Input: part model. Units: mm. Frame: model coordinates. Face numbers are marked on the shaded views. A direction names the side the tool comes from. Coordinates: 2 decimals unless noted, no trailing zeros. Order: outer loops, then holes, each group sorted by start corner. A loop starts at its lowest first (then second) coordinate and runs counter-clockwise, first axis right, second up.
from build123d import *

# Parameters (mm, degrees)
BOSS_EXTRUDE1_DEPTH = 54
BOSS_EXTRUDE2_DEPTH = 1.5
SKETCH3_W           = 2.3
SKETCH3_H           = 3
CUT_EXTRUDE1_DEPTH  = 0.5


with BuildPart() as part:
    # Sketch1 → Boss-Extrude1 (new body)
    with BuildSketch(Plane(origin=(0, 0, 0), x_dir=(0, 0, -1), z_dir=(1, 0, 0))):
        with BuildLine():
            Line((-15, 2.4), (15, 2.4))
            ThreePointArc((15, 2.4), (17.4, 0), (15, -2.4))
            Line((15, -2.4), (-15, -2.4))
            ThreePointArc((-15, -2.4), (-17.4, 0), (-15, 2.4))
        make_face()
    extrude(amount=BOSS_EXTRUDE1_DEPTH)

    # Sketch2 → Boss-Extrude2 (add)
    with BuildSketch(Plane(origin=(54, 0, 0), x_dir=(0, 0, -1), z_dir=(1, 0, 0))):
        with BuildLine():
            Line((-15, -2.6), (15, -2.6))
            ThreePointArc((15, -2.6), (17.6, 0), (15, 2.6))
            Line((15, 2.6), (-15, 2.6))
            ThreePointArc((-15, 2.6), (-17.6, 0), (-15, -2.6))
        make_face()
    extrude(amount=BOSS_EXTRUDE2_DEPTH)

    # Sketch3 → Cut-Extrude1 (cut)
    with BuildSketch(Plane(origin=(55.5, 0, 0), x_dir=(0, 0, -1), z_dir=(1, 0, 0))):
        with Locations((-12.85, 0)):
            Rectangle(SKETCH3_W, SKETCH3_H)
        with Locations((-9.85, 0)):
            Rectangle(SKETCH3_W, SKETCH3_H)
        with Locations((9.85, 0)):
            Rectangle(SKETCH3_W, SKETCH3_H)
        with Locations((12.85, 0)):
            Rectangle(SKETCH3_W, SKETCH3_H)
    extrude(amount=-CUT_EXTRUDE1_DEPTH, mode=Mode.SUBTRACT)


solid = part.part
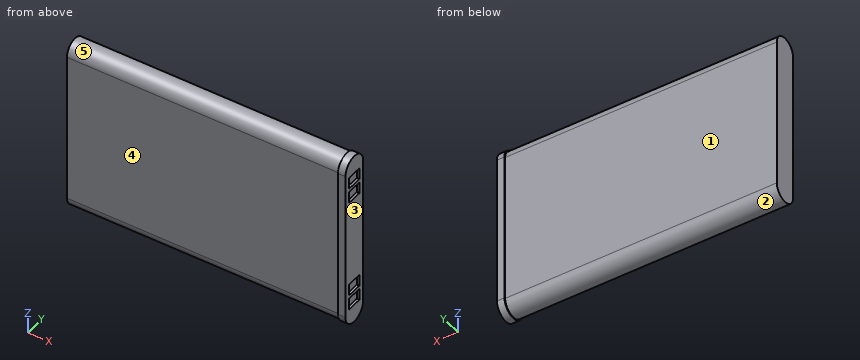
Item 1: Pin query (flat end, axial travel): pin 1 Ø2.5 at (y, z) = (-0.5, -13) entering from +X; pin 2 Ø0.6 at (x, y) = (55.5, -0.5) entering from -Z; pin 3 Ø1.2 at (y, z) = (0, 10) entering from +X; pin 4 Ø2 at (x, z) = (29.5, -7.5) entering from +Y. Return the tip coordinate at first contact, or that it passes through.
Response values:
pin 1: stops at x = 55.5
pin 2: stops at z = -17.59
pin 3: stops at x = 55
pin 4: stops at y = 2.4
Item 2: Cut plane B-B on x = 6.5. Return loops of the section in (y, z).
Response values:
outline: (-2.4, -15) arc R2.4 ccw to (2.4, -15) - (2.4, 15) arc R2.4 ccw to (-2.4, 15) - close
Item 3: Access query for the marked faces 1, 2, 3, 4 and 5. Directions: +Z, -Z, +X, -X, +Y, -Y. A direction counts if a zero-diameter tool reaches every point of the face in a straight line with its end or side. Return the directions, or none.
Response values:
face 1: +Z, -Z, -X, +Y
face 2: -Z, -X
face 3: +Z, -Z, +X, +Y, -Y
face 4: +Z, -Z, -X, -Y
face 5: +Z, -X
Item 4: Cut plane A-A on z = -9.5. Return loops of the section in (x, y), then the cut area to 4 significant figures.
Response values:
outline: (0, -2.4) - (54, -2.4) - (54, -2.6) - (55.5, -2.6) - (55.5, -1.5) - (55, -1.5) - (55, 1.5) - (55.5, 1.5) - (55.5, 2.6) - (54, 2.6) - (54, 2.4) - (0, 2.4) - close
area: 265.5 mm2
Item 5: Ray query, probe 1 along X at (y, z) = (1.25, 10); probe 2 along Y at (x, z) = (44, -1.5); probe 3 along Z at (x, y) = (45.5, 0.2). Return the intervals inside material, ascending.
Response values:
probe 1: x = 0 to 55
probe 2: y = -2.4 to 2.4
probe 3: z = -17.39 to 17.39
